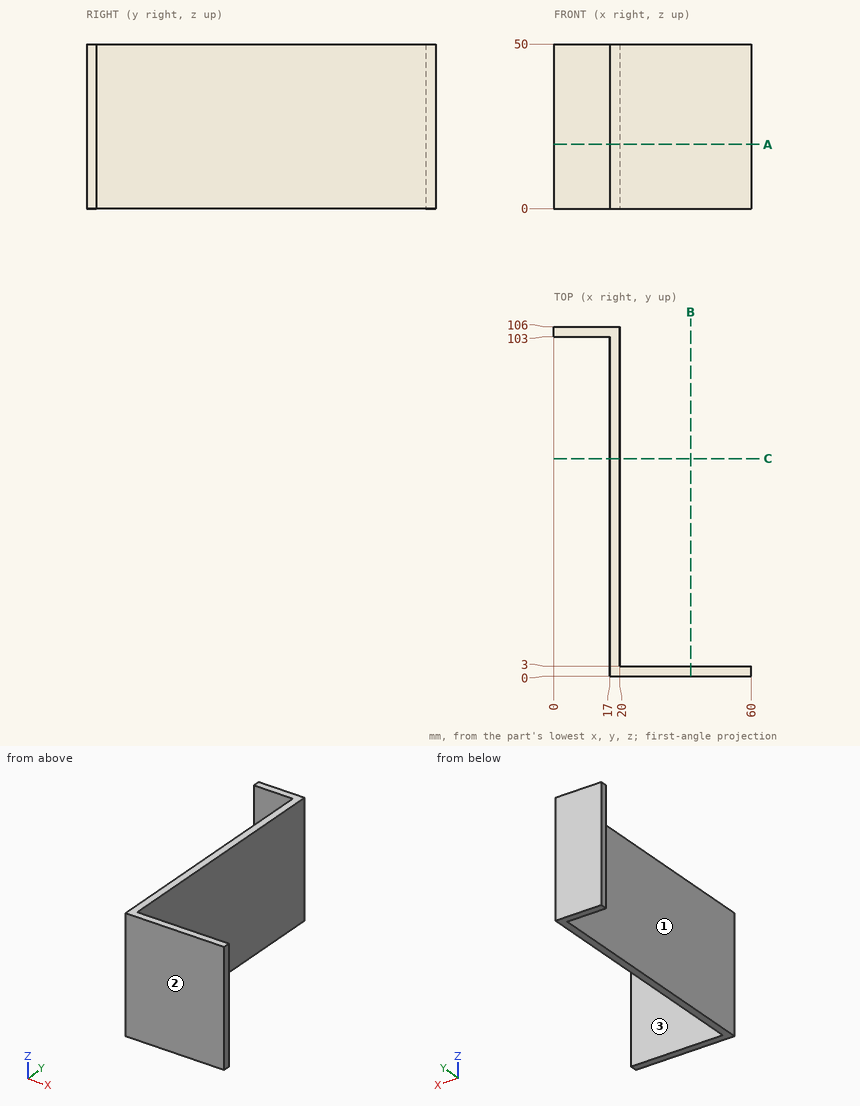
Geometry check sheet. Reference: drawing and pictorial views, mm from the part's lowest x, y, z. A direction names the side the tool comes from. Coordinates: 2 decimals unless noted, no trailing zeros. Loops run counter-clockwise (first coordinate to the right, second up) from the corner with the lowest first, then second, coordinate; pieces in that order, holes last. Notation, with made-up numbers: (25.25, 18.25) -> (77.25, 18.25) arc R22 ccw to (77.25, 37.25) -> close; hole circle Ø11 at (40.25, -27.5). An arc over 180 degrees is marked (long way). Put each result on its own line as item: value.
1) Cross-section at C-C on y = 66. Record the boundary of the cut face in (x, z), plus the area to 3 significant figures.
Result set:
outline: (17, 0) -> (20, 0) -> (20, 50) -> (17, 50) -> close
area: 150 mm^2
2) Cross-section at B-B on x = 41.5. Record the boundary of the cut face in (y, z), plus the area to 3 significant figures.
Result set:
outline: (0, 0) -> (3, 0) -> (3, 50) -> (0, 50) -> close
area: 150 mm^2
3) Cross-section at A-A on z = 19.5. Record the boundary of the cut face in (x, y), plus the area to 3 significant figures.
Result set:
outline: (0, 103) -> (17, 103) -> (17, 0) -> (60, 0) -> (60, 3) -> (20, 3) -> (20, 106) -> (0, 106) -> close
area: 489 mm^2
4) Gauge pin test, flat ends, axial feed: pin 1 Ø8 at (y, z) = (13, 31.5) entering from +X; pin 2 Ø12 at (y, z) = (89.5, 11.5) entering from -X; pin 3 Ø6 at (x, z) = (40, 24) entering from +Y. Record the tip position at first contact, or that the pin passes through.
Result set:
pin 1: stops at x = 20
pin 2: stops at x = 17
pin 3: stops at y = 3
5) Tool access check on the marked faces 1, 2 and 3. Record the directions out of +Z, -Z, +X, -X, +Y, -Y that give a thin tool (end or side, any length) a straight path to the whole face; none if there is none.
Result set:
face 1: +Z, -Z, -X, -Y
face 2: +Z, -Z, +X, -X, -Y
face 3: +Z, -Z, +X, +Y
6) Thickness scan on line 1 (X direction, y = 95.5, z = 16.5); line 2 (Y direction, x = 12, z = 17); line 3 (Y direction, x = 21.5, z = 25). Record the ranges inside material, lowest first.
Result set:
line 1: x = 17 to 20
line 2: y = 103 to 106
line 3: y = 0 to 3
